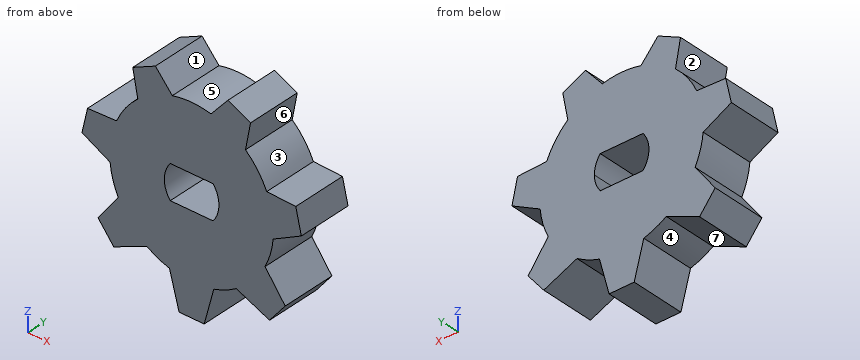
```python
from build123d import *

# Parameters (mm, degrees)
SKIZZE1_R                       = 7.5
AUFSATZ_LINEAR_AUSTRAGEN1_DEPTH = 5
AUFSATZ_LINEAR_AUSTRAGEN2_DEPTH = 5
KREISMUSTER1_COUNT              = 7
SCHNITT_LINEAR_AUSTRAGEN1_DEPTH = 5


with BuildPart() as part:
    # Skizze1 → Aufsatz-Linear austragen1 (new body)
    with BuildSketch(Plane(origin=(0, 0, 0), x_dir=(1, 0, 0), z_dir=(0, 1, 0))):
        with Locations(Location((0, 0, 0), (0, 0, 270))):
            Circle(SKIZZE1_R)
    extrude(amount=AUFSATZ_LINEAR_AUSTRAGEN1_DEPTH)

    # Skizze2 → Aufsatz-Linear austragen2 (add)
    with BuildSketch(Plane(origin=(0, 5, 0), x_dir=(1, 0, 0), z_dir=(0, 1, 0))):
        Polygon((-1.15, 10.5), (1.15, 10.5), (2.087822174, 7), (-2.087822174, 7), align=None)
    aufsatz_linear_austragen2 = extrude(amount=-AUFSATZ_LINEAR_AUSTRAGEN2_DEPTH)

    # Kreismuster1: Aufsatz-Linear austragen2 ×7 about axis
    kreismuster1_axis = Axis((0, 0, -0.45727081), (0, 1, 0))
    for i in range(1, KREISMUSTER1_COUNT):
        add(aufsatz_linear_austragen2.rotate(kreismuster1_axis, i * 360 / KREISMUSTER1_COUNT))

    # Skizze3 → Schnitt-Linear austragen1 (cut)
    with BuildSketch(Plane(origin=(0, 5, 0), x_dir=(1, 0, 0), z_dir=(0, 1, 0))):
        with BuildLine():
            Line((1.961504525, 1.55), (-1.961504525, 1.55))
            ThreePointArc((-1.961504525, 1.55), (-2.5, 0), (-1.961504525, -1.55))
            Line((-1.961504525, -1.55), (1.961504525, -1.55))
            ThreePointArc((1.961504525, -1.55), (2.361542008, -0.820438507), (2.5, 0))
            ThreePointArc((2.5, 0), (2.361542008, 0.820438507), (1.961504525, 1.55))
        make_face()
    extrude(amount=-SCHNITT_LINEAR_AUSTRAGEN1_DEPTH, mode=Mode.SUBTRACT)


solid = part.part
```
CAD build for the part. Positions are in the model's coordinates, mm. Face numbers are marked on the shaded views. A direction names the side the tool comes from. Round coordinates to 2 decimals unless told otherwise and drop trailing zeros. Order: outer loops, then holes, each group sorted by start corner. A loop starts at its lowest first (then second) coordinate and runs counter-clockwise, first axis right, second up.
Item 1: Mould opens along Z. For the marked faces 5, 6 and 7 say: pulls with the +Z half, pulls with the -Z half, needs draft (parallel to the pull), parting line crosses it, or undercut.
Item 2: Saw through at B-B on x = 7.75. Write the cut outline in (y, z).
Item 3: Pin check, flat tips, straight feed: pin 1 (1.2 mm diameter, centred on x = 0, y = 3.5, fed in from +Z); pin 2 (2 mm diameter, centred on y = 2, z = -0.5, fed in from -X). Stop position of each tip, or through.
Item 4: Tool access for the marked faces 1, 2, 3 and 4: list every direction of +Z, -Z, +X, -X, +Y, -Y with a clear straight run to the whole face (end or side of a thin tool).
Item 5: Saw through at D-D on z = 3.25. Write the cut outline in (x, y), then the cut area to 3 significant figures.
Item 6: Saw through at C-C on z = -8. Write the cut outline in (x, y), then the cut area to 3 significant figures.
Item 7: Probe line 1 along X through (y, z) = (2, -7.25); line 2 along X through (y, z) = (1.3, 7.75); line 3 along X through (y, z) = (0.95, -1.5). List the from-to ranges inside material, lowest first.
Reported:
1. face 5: pulls with the +Z half
1. face 6: undercut
1. face 7: pulls with the -Z half
2. outline: (0, -6.85) - (5, -6.85) - (5, -4.71) - (0, -4.71) - close; (0, -0.56) - (5, -0.56) - (5, 2.97) - (0, 2.97) - close
3. pin 1: stops at z = 7.5
3. pin 2: stops at x = -9.75
4. face 1: +Z, +Y, -Y
4. face 2: -X, +Y, -Y
4. face 3: +X, +Y, -Y
4. face 4: -Z, +Y, -Y
5. outline: (-6.76, 0) - (6.76, 0) - (6.76, 5) - (-6.76, 5) - close
5. area: 67.6 mm2
6. outline: (-1.82, 0) - (1.82, 0) - (1.82, 5) - (-1.82, 5) - close
6. area: 18.2 mm2
7. line 1: x = -7.43 to -6.29, -2.02 to 2.02, 6.29 to 7.43
7. line 2: x = -5.33 to -2.17, 2.17 to 5.33
7. line 3: x = -7.35 to -2, 2 to 7.35
